Source: CAD feature listing. Evaluate the final solid. Frame: model axes, mm. A direction names the side the tool comes from. Give positions to 0.01 mm unless a question says otherwise; leave off trailing zeros. Loops run counter-clockwise (first coordinate to the right, second up) from the corner with the lowest first, then second, coordinate; pieces in that order, holes last. Notation, with made-up numbers: (73, -16.5) - (80, -16.5) arc R23 cw to (80, -4.5) - close; hole circle Ø1 at (60, -31). An arc over 180 degrees is marked (long way). Write each question's results on one line, items separated by ' | '. Start each with the question number.
(1) Cut plane C-C on y = 2.5. Return the cut outline in (x, z).
(2) Contact query for flat-ended pins moving along their axis: pin 1 (1.5 mm diameter, centred on y = 13, z = 1.5, fed in from -X); pin 2 (9 mm diameter, centred on x = -9.5, y = -1.5, fed in from +Z); pin 3 (1.2 mm diameter, centred on y = -1, z = 2.5, fed in from +X). Output: stop coordinate, or through.
(3) Reachability of faces 1 (the flat face through (12, 5, 3)), 2 (the flat face through (-14.303, -9.283, 2.972)), 3 (the flat face through (9.911, 5.683, 0.526)), 4 (the flat face through (14.5, -2.6, 0.5)) from +Z, -Z, +X, -X, +Y, -Y: full face, straight path, thin tool, end or side. Return the list, or none.
(4) Cut plane B-B on x = -10. Return the cut outline in (y, z).
(5) Cut plane A-A on y = -5.2. Return the cut outline in (x, z).
(6) Material intervals for line 1 along Y through (x, z) = (-10, 1.6); line 2 along X through (y, z) = (-4, 3.25); line 3 along X through (y, z) = (-5, 1.25), sorted ascending. Write a range as [from, to].
from build123d import *

# Parameters (mm, degrees)
SKETCH002_R     = 4.75
SKETCH_R        = 1.6
PAD_DEPTH       = 5
PAD001_DEPTH    = 2.5
SKETCH004_R     = 6
POCKET_DEPTH    = 14
FILLET_R        = 1
FILLET001_R     = 1
CHAMFER_SIZE    = 1
CHAMFER001_SIZE = 0.25
FILLET002_R     = 0.5
FILLET003_R     = 0.3


with BuildPart() as sweep_body:
    # Sweep: sweep along a path in Sketch003
    with BuildLine(Plane.XY.offset(7.5)) as sweep_path:
        Line((14.142136, 19.242641), (0, 5.100505))
        Line((0, 5.100505), (0, -5.899495))
    # Sketch002 → Sweep (sweep)
    with BuildSketch(Plane(origin=(15.763456, 15.763456, 0), x_dir=(-0.707107, 0.707107, 0), z_dir=(0.707107, 0.707107, 0))):
        with Locations((3.606602, 7.5)):
            Circle(SKETCH002_R)
    sweep(path=sweep_path.line, transition=Transition.RIGHT)


with BuildPart() as fillet003:
    # Sketch → Pad (new body)
    with BuildSketch(Plane.XY):
        Polygon((-15, 3.585786), (-15, -8.585786), (-13.585786, -10), (13.585786, -10), (15, -8.585786), (15, 3.585786), (13.585786, 5), (10.384776, 5), (10.384776, 7), (17.455844, 14.071068), (8.970563, 22.556349), (-8.585786, 5), (-13.585786, 5), align=None)
        with Locations((-10, -5.2)):
            Circle(SKETCH_R, mode=Mode.SUBTRACT)
        with Locations((10, -5.2)):
            Circle(SKETCH_R, mode=Mode.SUBTRACT)
    extrude(amount=PAD_DEPTH)

    # Sketch001 → Pad001 (new body)
    with BuildSketch(Plane.XY.offset(5)):
        Polygon((-8.585786, 5), (8.970563, 22.556349), (17.455844, 14.071068), (10.384776, 7), (10.384776, 5), align=None)
    extrude(amount=PAD001_DEPTH)

    # Cut: cut Sweep body
    add(sweep_body.part, mode=Mode.SUBTRACT)

    # Sketch004 → Pocket (cut)
    with BuildSketch(Plane.XZ.offset(10)):
        with Locations((0, 7.5)):
            Circle(SKETCH004_R)
    extrude(amount=-POCKET_DEPTH, mode=Mode.SUBTRACT)

    # Fillet
    fillet_edges = [fillet003.edges().sort_by_distance(p)[0] for p in [
        (-0.997031, 4, 2.855818),
    ]]
    fillet(fillet_edges, radius=FILLET_R)

    # Fillet001
    fillet001_edges = [fillet003.edges().sort_by_distance(p)[0] for p in [
        (-4.568761, 5, 6.200413),
    ]]
    fillet(fillet001_edges, radius=FILLET001_R)

    # Chamfer
    chamfer_edges = [fillet003.edges().sort_by_distance(p)[0] for p in [
        (0, -10, 0),
        (14.292893, -9.292893, 0),
        (15, -2.5, 0),
        (11.985281, 5, 0),
        (14.292893, 4.292893, 0),
        (10.384776, 6, 0),
        (13.92031, 10.535534, 0),
        (13.213203, 18.313708, 0),
        (0.192388, 13.778175, 0),
        (-11.085786, 5, 0),
        (-14.292893, 4.292893, 0),
        (-15, -2.5, 0),
        (-14.292893, -9.292893, 0),
    ]]
    chamfer(chamfer_edges, length=CHAMFER_SIZE)

    # Chamfer001
    chamfer001_edges = [fillet003.edges().sort_by_distance(p)[0] for p in [
        (-11.6, -5.2, 0),
        (8.4, -5.2, 0),
    ]]
    chamfer(chamfer001_edges, length=CHAMFER001_SIZE)

    # Fillet002
    fillet002_edges = [fillet003.edges().sort_by_distance(p)[0] for p in [
        (10.384776, 5, 6.25),
        (10.384776, 7, 4.25),
        (-8.585786, 5, 6.25),
    ]]
    fillet(fillet002_edges, radius=FILLET002_R)

    # Fillet003
    fillet003_edges = [fillet003.edges().sort_by_distance(p)[0] for p in [
        (6.343838, 5, 6.159209),
    ]]
    fillet(fillet003_edges, radius=FILLET003_R)


solid = fillet003.part
Ans:
1) outline: (-15, 1) - (-14, 0) - (14, 0) - (15, 1) - (15, 5) - (5.45, 5) arc R6 cw to (-5.45, 5) - (-15, 5) - close
2) pin 1: x = -1.34 | pin 2: z = 5 | pin 3: x = 15
3) face 1: +Z, -Z, +X | face 2: +Z, -Z, -X, -Y | face 3: -Z, +X | face 4: -Z, +X, -Y
4) outline: (-10, 1) - (-9, 0) - (-7.05, 0) - (-6.8, 0.25) - (-6.8, 5) - (-10, 5) - close; (-3.6, 0.25) - (-3.35, 0) - (4, 0) - (5, 1) - (5, 5) - (-3.6, 5) - close
5) outline: (-15, 1) - (-14, 0) - (-11.85, 0) - (-11.6, 0.25) - (-11.6, 5) - (-15, 5) - close; (-8.4, 0.25) - (-8.15, 0) - (8.15, 0) - (8.4, 0.25) - (8.4, 5) - (5.45, 5) arc R6 cw to (-5.45, 5) - (-8.4, 5) - close; (11.6, 0.25) - (11.85, 0) - (14, 0) - (15, 1) - (15, 5) - (11.6, 5) - close
6) line 1: [-10, -6.8], [-3.6, 5] | line 2: [-15, -11.06], [-8.94, -4.24], [4.24, 8.94], [11.06, 15] | line 3: [-15, -11.59], [-8.41, 8.41], [11.59, 15]
